Geometry: final body of the model. Coordinates: model frame, mm. A direction names the side the tool comes from. Give positions to 0.01 mm unless a question says otherwise; leave off trailing zeros. Order: outer loops, then holes, each group sorted by start corner. A loop starts at its lowest first (then second) coordinate and runs counter-clockwise, first axis right, second up. Notation, with made-up numbers: (25.25, -39) -> (48.25, -39) arc R20 ccw to (48.25, -8) -> close; hole circle Ø8 at (56.25, -21). An arc over 180 degrees is marked (long way). One line per item, written item: value. Start each with the question number.
```python
from build123d import *

# Parameters (mm, degrees)
SKETCH1_R               = 55
BOSS_EXTRUDE1_DEPTH     = 3
SKETCH2_W               = 90
SKETCH2_H               = 140
BOSS_EXTRUDE2_DEPTH     = 3
SKETCH4_R               = 46
CUT_EXTRUDE2_DEPTH      = 1
CUT_EXTRUDE2_DEPTH_BACK = 4
CUT_EXTRUDE5_START      = -4
CUT_EXTRUDE5_DEPTH      = 5
CUT_EXTRUDE3_START      = -4
SKETCH5_R               = 2.25
CUT_EXTRUDE3_DEPTH      = 5
CIRPATTERN1_COUNT       = 12
CUT_EXTRUDE4_START      = -4
SKETCH6_R               = 4.25
CUT_EXTRUDE4_DEPTH      = 5
LPATTERN1_COUNT         = 3
LPATTERN1_PITCH         = 20


with BuildPart() as part:
    # Sketch1 → Boss-Extrude1 (new body)
    with BuildSketch(Plane(origin=(0, 0, 0), x_dir=(1, 0, 0), z_dir=(0, 1, 0))):
        Circle(SKETCH1_R)
    extrude(amount=BOSS_EXTRUDE1_DEPTH)

    # Sketch2 → Boss-Extrude2 (add)
    with BuildSketch(Plane(origin=(0, 0, 0), x_dir=(1, 0, 0), z_dir=(0, 1, 0))):
        with Locations((0, 101.622776602)):
            Rectangle(SKETCH2_W, SKETCH2_H)
    extrude(amount=BOSS_EXTRUDE2_DEPTH)

    # Sketch4 → Cut-Extrude2 (cut, two sides)
    with BuildSketch(Plane(origin=(0, 3, 0), x_dir=(1, 0, 0), z_dir=(0, 1, 0))) as cut_extrude2_sk:
        Circle(SKETCH4_R)
    extrude(amount=CUT_EXTRUDE2_DEPTH, mode=Mode.SUBTRACT)
    extrude(cut_extrude2_sk.sketch, amount=-CUT_EXTRUDE2_DEPTH_BACK, mode=Mode.SUBTRACT)

    # Sketch7 → Cut-Extrude5 (cut)
    with BuildSketch(Plane(origin=(0, 3, 0), x_dir=(1, 0, 0), z_dir=(0, 1, 0)).offset(CUT_EXTRUDE5_START)):
        with BuildLine():
            Line((0, 0), (0, -55))
            ThreePointArc((0, -55), (-24.969477486, -49.00535883), (-44.495934691, -32.328188876))
            Line((-44.495934691, -32.328188876), (0, 0))
        make_face()
    cut_extrude5 = extrude(amount=CUT_EXTRUDE5_DEPTH, mode=Mode.SUBTRACT)

    # Mirror1: Cut-Extrude5 across plane
    add(cut_extrude5.mirror(Plane(origin=(0, 0, 0), x_dir=(0, 0, 1), z_dir=(1, 0, 0))), mode=Mode.SUBTRACT)

    # Sketch5 → Cut-Extrude3 (cut)
    with BuildSketch(Plane(origin=(0, 3, 0), x_dir=(1, 0, 0), z_dir=(0, 1, 0)).offset(CUT_EXTRUDE3_START)):
        with Locations((0, 51)):
            Circle(SKETCH5_R)
    cut_extrude3 = extrude(amount=CUT_EXTRUDE3_DEPTH, mode=Mode.SUBTRACT)

    # CirPattern1: Cut-Extrude3 ×12 about axis
    cirpattern1_axis = Axis((0, 0, 0), (0, 1, 0))
    for i in range(1, CIRPATTERN1_COUNT):
        add(cut_extrude3.rotate(cirpattern1_axis, i * 360 / CIRPATTERN1_COUNT), mode=Mode.SUBTRACT)

    # Sketch6 → Cut-Extrude4 (cut)
    with BuildSketch(Plane(origin=(0, 3, 0), x_dir=(1, 0, 0), z_dir=(0, 1, 0)).offset(CUT_EXTRUDE4_START)):
        with Locations((20, 151.622776602)):
            Circle(SKETCH6_R)
        with Locations((-20, 151.622776602)):
            Circle(SKETCH6_R)
    cut_extrude4 = extrude(amount=CUT_EXTRUDE4_DEPTH, mode=Mode.SUBTRACT)

    # LPattern1: Cut-Extrude4 ×3
    with Locations(*[(0, 0, i * LPATTERN1_PITCH) for i in range(1, LPATTERN1_COUNT)]):
        add(cut_extrude4, mode=Mode.SUBTRACT)


solid = part.part
```
1. Cut plane D-D, the plane x = -20.5. Return loops of the section in (y, z).
2. Cut plane C-C, the plane z = -51. Return loops of the section in (x, y), then the cut area to 4 significant figures.
3. Cut plane A-A, the plane z = 0. Return loops of the section in (x, y), then the cut area to 3 significant figures.
4. Material intervals for L1, parallel to X at y = 2.45, z = -152; L2, parallel to X at y = 1.95, z = 0; L3, parallel to Z at x = 20, y = 0.8, sorted ascending. Write a range as [from, to].
5. Cut plane B-B, the plane x = 0. Return loops of the section in (y, z).
6. Pin query (flat end, axial travel): P1, Ø1.5, axis at y = 0.5, z = -47, coming from the -X side. Return the tip coordinate at first contact, or that it passes through.
7. Draft query along X for faces 3 (the cylindrical face through (54.992, 1.479, 0.911)), 4 (the flat face through (-1, 3, -94)), 5 (the cylindrical face through (-0.29, 1.48, -53.23)). Return one class per face: pulls with the +X half, pulls with the -X half, needs draft (parallel to the pull), parting line crosses it, or undercut.
8. Access query for faces 1 (the cylindrical face through (19.079, 1.479, -147.474)), 2 (the flat face through (-40.906, 1.479, 29.72)). Directions: +Z, -Z, +X, -X, +Y, -Y. A direction counts if a zero-diameter tool reaches every point of the face in a straight line with its end or side. Return the directions, or none.
Answers follow:
1. outline: (0, -171.62) -> (3, -171.62) -> (3, -155.84) -> (0, -155.84) -> close; (0, -147.4) -> (3, -147.4) -> (3, -135.84) -> (0, -135.84) -> close; (0, -127.4) -> (3, -127.4) -> (3, -115.84) -> (0, -115.84) -> close; (0, -107.4) -> (3, -107.4) -> (3, -41.18) -> (0, -41.18) -> close
2. outline: (-45, 0) -> (-2.25, 0) -> (-2.25, 3) -> (-45, 3) -> close; (2.25, 0) -> (45, 0) -> (45, 3) -> (2.25, 3) -> close
2. area: 256.5 mm²
3. outline: (-55, 0) -> (-53.25, 0) -> (-53.25, 3) -> (-55, 3) -> close; (-48.75, 0) -> (-46, 0) -> (-46, 3) -> (-48.75, 3) -> close; (46, 0) -> (48.75, 0) -> (48.75, 3) -> (46, 3) -> close; (53.25, 0) -> (55, 0) -> (55, 3) -> (53.25, 3) -> close
3. area: 27.0 mm²
4. L1: x = [-45, -24.23], [-15.77, 15.77], [24.23, 45]
4. L2: x = [-55, -53.25], [-48.75, -46], [46, 48.75], [53.25, 55]
4. L3: z = [-171.62, -155.87], [-147.37, -135.87], [-127.37, -115.87], [-107.37, -41.42]
5. outline: (0, -171.62) -> (3, -171.62) -> (3, -53.25) -> (0, -53.25) -> close; (0, -48.75) -> (3, -48.75) -> (3, -46) -> (0, -46) -> close
6. P1: stops at x = -45
7. face 3: pulls with the +X half
7. face 4: needs draft
7. face 5: undercut
8. face 1: +Y, -Y
8. face 2: +Z, +Y, -Y
